For this review, take the finished solid that the model builds, in its own axes (mm). A direction names the side the tool comes from. Round coordinates to 2 decimals unless told otherwise and drop trailing zeros. Order: outer loops, then holes, each group sorted by start corner. A loop starts at its lowest first (then second) coordinate and runs counter-clockwise, first axis right, second up.
from build123d import *

# Parameters (mm, degrees)
SKETCH1_W                = 25
SKETCH1_H                = 25
BOSS_EXTRUDE1_DEPTH      = 2
BOSS_EXTRUDE2_DEPTH      = 15
BOSS_EXTRUDE2_DEPTH_BACK = 2
SKETCH2_W                = 25
SKETCH2_H                = 2
SKETCH3_R                = 2.025
CUT_EXTRUDE1_DEPTH       = 35.960692213
FILLET1_R                = 2
FILLET2_R                = 1
SKETCH4_W                = 21
SKETCH4_H                = 2
BOSS_EXTRUDE3_DEPTH      = 3
SKETCH5_W                = 21
SKETCH5_H                = 2
BOSS_EXTRUDE4_DEPTH      = 15
BOSS_EXTRUDE5_DEPTH      = 15
BOSS_EXTRUDE5_DEPTH_BACK = 36
SKETCH6_W                = 10
SKETCH6_H                = 2
SKETCH7_W                = 2
SKETCH7_H                = 41
BOSS_EXTRUDE6_DEPTH      = 105
SKETCH8_W                = 10
SKETCH8_H                = 4
CUT_EXTRUDE2_DEPTH       = 118.389309564
FILLET3_R                = 1
FILLET4_R                = 2
CUT_EXTRUDE3_DEPTH       = 119.102709537
SKETCH12_R               = 7.025
CUT_EXTRUDE4_DEPTH       = 119.102709537
CUT_EXTRUDE5_DEPTH       = 119.102709537
FILLET7_R                = 6
FILLET8_R                = 6
SKETCH14_W               = 10
SKETCH14_H               = 5
CUT_EXTRUDE6_DEPTH       = 112.496636721


with BuildPart() as part:
    # Sketch1 → Boss-Extrude1 (new body)
    with BuildSketch(Plane(origin=(0, 0, 0), x_dir=(1, 0, 0), z_dir=(0, 1, 0))):
        Rectangle(SKETCH1_W, SKETCH1_H)
    extrude(amount=BOSS_EXTRUDE1_DEPTH)

    # Sketch2 → Boss-Extrude2 (add, two sides: drawn at the far end of the back side and taken through both)
    with BuildSketch(Plane.XZ.offset(-BOSS_EXTRUDE2_DEPTH_BACK)):
        with Locations((0, 13.5)):
            Rectangle(SKETCH2_W, SKETCH2_H)
        with Locations((0, -13.5)):
            Rectangle(SKETCH2_W, SKETCH2_H)
    extrude(amount=BOSS_EXTRUDE2_DEPTH + BOSS_EXTRUDE2_DEPTH_BACK)

    # Sketch3 → Cut-Extrude1 (cut, through all)
    with BuildSketch(Plane.XY.offset(14.5)):
        with Locations((-9.5, -10)):
            Circle(SKETCH3_R)
        with Locations((5.5, -10)):
            Circle(SKETCH3_R)
    extrude(amount=-CUT_EXTRUDE1_DEPTH, mode=Mode.SUBTRACT)

    # Fillet1
    fillet1_edges = [part.edges().sort_by_distance(p)[0] for p in [
        (0, 2, 14.5),
        (0, 2, -14.5),
    ]]
    fillet(fillet1_edges, radius=FILLET1_R)

    # Fillet2
    fillet2_edges = [part.edges().sort_by_distance(p)[0] for p in [
        (0, 0, 12.5),
        (0, 0, -12.5),
    ]]
    fillet(fillet2_edges, radius=FILLET2_R)

    # Sketch4 → Boss-Extrude3 (add)
    with BuildSketch(Plane.ZY.offset(12.5)):
        with Locations((0, 1)):
            Rectangle(SKETCH4_W, SKETCH4_H)
    extrude(amount=BOSS_EXTRUDE3_DEPTH)

    # Sketch5 → Boss-Extrude4 (add)
    with BuildSketch(Plane(origin=(12.5, 0, 0), x_dir=(0, 0, -1), z_dir=(1, 0, 0))):
        with Locations((0, 1)):
            Rectangle(SKETCH5_W, SKETCH5_H)
    extrude(amount=BOSS_EXTRUDE4_DEPTH)

    # Sketch6 → Boss-Extrude5 (add, two sides: drawn at the far end of the back side and taken through both)
    with BuildSketch(Plane.XY.offset(10.5).offset(-BOSS_EXTRUDE5_DEPTH_BACK)):
        with Locations((22.5, 1)):
            Rectangle(SKETCH6_W, SKETCH6_H)
    extrude(amount=BOSS_EXTRUDE5_DEPTH + BOSS_EXTRUDE5_DEPTH_BACK)

    # Sketch7 → Boss-Extrude6 (add)
    with BuildSketch(Plane(origin=(0, 2, 0), x_dir=(1, 0, 0), z_dir=(0, 1, 0))):
        with Locations((-14.5, 0)):
            Rectangle(SKETCH7_W, SKETCH7_H)
    extrude(amount=BOSS_EXTRUDE6_DEPTH)

    # Sketch8 → Cut-Extrude2 (cut, through all)
    with BuildSketch(Plane(origin=(-13.5, 0, 0), x_dir=(0, 0, -1), z_dir=(1, 0, 0))):
        with Locations((-15.5, 4)):
            Rectangle(SKETCH8_W, SKETCH8_H)
        with Locations((15.5, 4)):
            Rectangle(SKETCH8_W, SKETCH8_H)
    extrude(amount=-CUT_EXTRUDE2_DEPTH, mode=Mode.SUBTRACT)

    # Fillet3
    fillet3_edges = [part.edges().sort_by_distance(p)[0] for p in [
        (-13.5, 2, 0),
    ]]
    fillet(fillet3_edges, radius=FILLET3_R)

    # Fillet4
    fillet4_edges = [part.edges().sort_by_distance(p)[0] for p in [
        (-15.5, 0, 0),
    ]]
    fillet(fillet4_edges, radius=FILLET4_R)

    # Sketch10 → Cut-Extrude3 (cut, through all)
    with BuildSketch(Plane.ZY.offset(15.5)):
        with BuildLine():
            Line((11.5, 56), (11.5, 26))
            ThreePointArc((11.5, 26), (0, 14.5), (-11.5, 26))
            Line((-11.5, 26), (-11.5, 56))
            ThreePointArc((-11.5, 56), (0, 67.5), (11.5, 56))
        make_face()
        with BuildLine():
            Line((-12.4975, 56), (-12.4975, 26))
            ThreePointArc((-12.4975, 26), (-14, 24.4975), (-15.5025, 26))
            Line((-15.5025, 26), (-15.5025, 56))
            ThreePointArc((-15.5025, 56), (-14, 57.5025), (-12.4975, 56))
        make_face()
        with BuildLine():
            Line((12.4975, 56), (12.4975, 26))
            ThreePointArc((12.4975, 26), (14, 24.4975), (15.5025, 26))
            Line((15.5025, 26), (15.5025, 56))
            ThreePointArc((15.5025, 56), (14, 57.5025), (12.4975, 56))
        make_face()
    extrude(amount=-CUT_EXTRUDE3_DEPTH, mode=Mode.SUBTRACT)

    # Sketch12 → Cut-Extrude4 (cut, through all)
    with BuildSketch(Plane.ZY.offset(15.5)):
        with Locations((0, 97)):
            Circle(SKETCH12_R)
    extrude(amount=-CUT_EXTRUDE4_DEPTH, mode=Mode.SUBTRACT)

    # Sketch13 → Cut-Extrude5 (cut, through all)
    with BuildSketch(Plane.ZY.offset(15.5)):
        Polygon((-20.5, 107), (-20.5, 67), (-12.5, 75), (-12.5, 107), align=None)
        Polygon((12.5, 75), (12.5, 107), (20.5, 107), (20.5, 67), align=None)
    extrude(amount=-CUT_EXTRUDE5_DEPTH, mode=Mode.SUBTRACT)

    # Fillet7
    fillet7_edges = [part.edges().sort_by_distance(p)[0] for p in [
        (-14.5, 107, 12.5),
        (-14.5, 107, -12.5),
    ]]
    fillet(fillet7_edges, radius=FILLET7_R)

    # Fillet8
    fillet8_edges = [part.edges().sort_by_distance(p)[0] for p in [
        (-14.5, 6, 20.5),
        (-14.5, 6, -20.5),
    ]]
    fillet(fillet8_edges, radius=FILLET8_R)

    # Sketch14 → Cut-Extrude6 (cut, through all)
    with BuildSketch(Plane(origin=(0, 2, 0), x_dir=(1, 0, 0), z_dir=(0, 1, 0))):
        with Locations((22.5, 23)):
            Rectangle(SKETCH14_W, SKETCH14_H)
        with Locations((22.5, -23)):
            Rectangle(SKETCH14_W, SKETCH14_H)
    extrude(amount=-CUT_EXTRUDE6_DEPTH, mode=Mode.SUBTRACT)


solid = part.part
(1) Wall thickness on L1, parallel to X at y = 73, z = 4; L2, parallel to Y at x = -6, z = -5.5; L3, parallel to Z at x = -11, y = -1.5: over which ranges is each line inside the solid? List them lowest first.
(2) Add section C-C on y = 32.5. Give the boundary of the cut face in (x, z).
(3) Tool access review of faces 1 (the face through (-14, 3, -10.5)), 2 (the face through (12, 2, 0)), 3 (the face through (-14, 3, 10.5)), 4 (the face through (12.5, -6, -13)): name each direction out of +Z, -Z, +X, -X, +Y, -Y from which nothing blocks a thin tool from reaching the whole face with its end or side.
(4) Add section B-B on x = 5.5. Give the boundary of the cut face in (y, z) (3 decimals), plus the area to 3 significant figures.
(5) Draft analysis for pull direction Y (two halves, no side actions). For faces 5 (the face through (-15.5, 65, -9)), 6 (the face through (-14.514, 103.965, -0.915)), 7 (the face through (-14.486, 105.289, 10.696)), state which applies: pulls with the +Y half, pulls with the -Y half, needs draft (parallel to the pull), parting line crosses it, or undercut.
(6) Add section D-D on z = -4. Give the boundary of the cut face in (x, y) (3 decimals).
(7) Clearance check with flat-ended pins moving along their axes: P1, Ø2.5, axis at x = -14.5, y = 3.5, coming from the -Z side; P2, Ø3, axis at y = -5, z = 12, coming from the -X side; P3, Ø1.2, axis at y = -10.5, z = -12, coming from the +X side. State where each tip first meets the part, or that it passes through.
(8) Add section A-A on y = -10. Give the boundary of the cut face in (x, z) (3 decimals), plus the area to 3 significant figures.
Here are the results:
1. L1: x = -15.5 to -13.5
1. L2: y = 0 to 2
1. L3: z = -14.5 to -12.5, 12.5 to 14.5
2. outline: (-15.5, -20.5) - (-13.5, -20.5) - (-13.5, -15.5) - (-15.5, -15.5) - close; (-15.5, -12.5) - (-13.5, -12.5) - (-13.5, -11.5) - (-15.5, -11.5) - close; (-15.5, 11.5) - (-13.5, 11.5) - (-13.5, 12.5) - (-15.5, 12.5) - close; (-15.5, 15.5) - (-13.5, 15.5) - (-13.5, 20.5) - (-15.5, 20.5) - close
3. face 1: -Z, -X, -Y
3. face 2: +Z, -Z, +X, +Y
3. face 3: +Z, -X, -Y
3. face 4: -Z, +Y, -Y
4. outline: (-15, -14.5) - (-12.025, -14.5) - (-12.025, -12.5) - (-15, -12.5) - close; (-15, 12.5) - (-12.025, 12.5) - (-12.025, 14.5) - (-15, 14.5) - close; (-7.975, -14.5) - (0, -14.5) arc R2 ccw to (2, -12.5) - (2, 12.5) arc R2 ccw to (0, 14.5) - (-7.975, 14.5) - (-7.975, 12.5) - (-1, 12.5) arc R1 cw to (0, 11.5) - (0, -11.5) arc R1 cw to (-1, -12.5) - (-7.975, -12.5) - close
4. area: 101 mm2
5. face 5: needs draft
5. face 6: undercut
5. face 7: pulls with the +Y half
6. outline: (-15.5, 2) arc R2 ccw to (-13.5, 0) - (27.5, 0) - (27.5, 2) - (-12.5, 2) arc R1 cw to (-13.5, 3) - (-13.5, 15.218) - (-15.5, 15.218) - close; (-15.5, 66.782) - (-13.5, 66.782) - (-13.5, 91.225) - (-15.5, 91.225) - close; (-15.5, 102.775) - (-13.5, 102.775) - (-13.5, 107) - (-15.5, 107) - close
7. P1: stops at z = -10.5
7. P2: stops at x = -12.5
7. P3: stops at x = 12.5
8. outline: (-12.5, -14.5) - (-11.525, -14.5) - (-11.525, -12.5) - (-12.5, -12.5) - close; (-12.5, 12.5) - (-11.525, 12.5) - (-11.525, 14.5) - (-12.5, 14.5) - close; (-7.475, -14.5) - (3.475, -14.5) - (3.475, -12.5) - (-7.475, -12.5) - close; (-7.475, 12.5) - (3.475, 12.5) - (3.475, 14.5) - (-7.475, 14.5) - close; (7.525, -14.5) - (12.5, -14.5) - (12.5, -12.5) - (7.525, -12.5) - close; (7.525, 12.5) - (12.5, 12.5) - (12.5, 14.5) - (7.525, 14.5) - close
8. area: 67.6 mm2
